Read the model definition and answer for the solid it produces. Units are mm, in the model's axes. Coordinates: 2 decimals unless noted, no trailing zeros. Write each loop counter-clockwise with the first axis right and the second up, starting at its lowest first coordinate (ties: lowest second). Pieces come first, ordered by that corner, then holes. Notation, with made-up numbers: (66.5, -18) -> (74.5, -18) arc R24 ccw to (74.5, 15) -> close; hole circle Ø9 at (21, 31.25). An arc over 180 degrees is marked (long way). Return JSON: item names as keys, results as strings.
from build123d import *

# Parameters (mm, degrees)
F3_DEPTH = 1000


with BuildPart() as f3:
    # F2 (on face) → F3 (new body)
    with BuildSketch(Plane.XY):
        with BuildLine():
            Line((303.86036, -165.789379), (491.060221, -165.560671))
            Line((491.060221, -165.560671), (490.9747, -95.560723))
            Line((490.9747, -95.560723), (0, 0))
            Line((0, 0), (-38.397282, -105.840393))
            ThreePointArc((-38.397282, -105.840393), (130.107793, -150.794242), (303.86036, -165.789379))
        make_face()
    extrude(amount=F3_DEPTH)


solid = f3.part
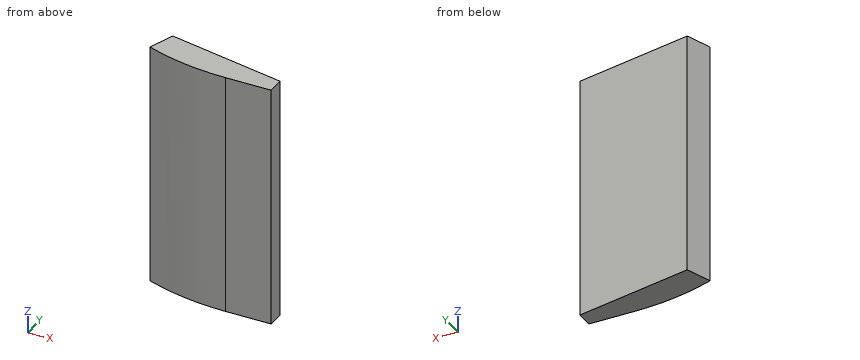
1. Consider L1, parallel to Y at x = 222, z = 365; L2, parallel to Y at x = 125.5, z = 808.5; L3, parallel to X at y = -105, z = 42. Determine where each line is inside the solid, lowest interval first.
Taken from the geometry:
{"L1": "y = -162.53 to -43.21", "L2": "y = -149.98 to -24.43", "L3": "x = -38.09 to 490.99"}
2. The part is cut by section B-B (x = 329.5). Determine the outline of the cut face in (y, z).
Taken from the geometry:
{"outline": "(-165.76, 0) -> (-64.13, 0) -> (-64.13, 1000) -> (-165.76, 1000) -> close"}
3. The part is cut by section A-A (z = 261). Determine the outline of the cut face in (x, y).
Taken from the geometry:
{"outline": "(-38.4, -105.84) arc R1000 ccw to (303.86, -165.79) -> (491.06, -165.56) -> (490.97, -95.56) -> (0, 0) -> close"}
4. The part is cut by section C-C (y = -127). Determine the outline of the cut face in (x, z).
Taken from the geometry:
{"outline": "(26.82, 0) -> (491.01, 0) -> (491.01, 1000) -> (26.82, 1000) -> close"}
5. Flat-ended cylindrical pins translate along their axes: pin 1 Ø3 at (y, z) = (-137, 748) entering from +X; pin 2 Ø5 at (y, z) = (-57.5, 624) entering from -X; pin 3 Ø1 at (x, z) = (358, 402) entering from -Y. Find the tip coordinate at first contact, or state that the pin passes through.
Taken from the geometry:
{"pin 1": "stops at x = 491.03", "pin 2": "stops at x = -21.77", "pin 3": "stops at y = -165.72"}
